Part print with two shaded views. Sizes in mm from the minimum x, y, z corner. Give positions to 0.01 mm unless a question says otherwise; leave off trailing zeros. Write each loop counter-clockwise with the first axis right and the second up, starting at its lowest first coordinate (ties: lowest second). Pieces come first, ordered by that corner, then holes. Notation, with made-up numbers: M -36,62.5 L 11,62.5 A36 ccw 11,101.5 Z; hole C -37,22.25 d6. An arc over 180 degrees is marked long. One line per item, written item: value. Start each with the question number.
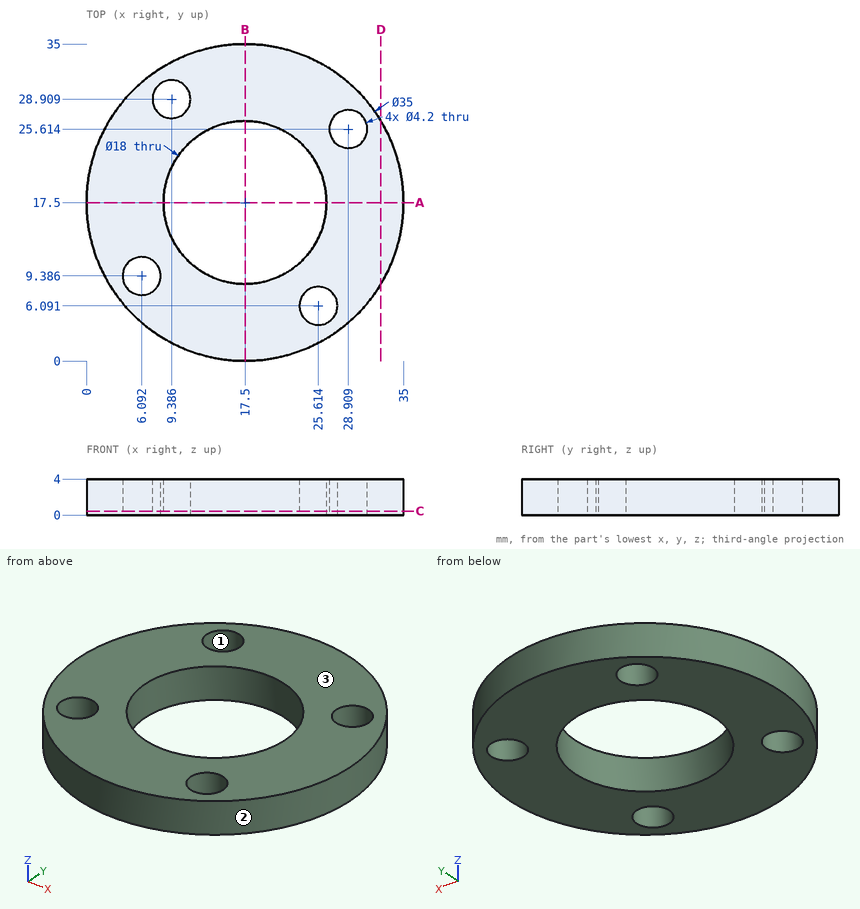
1) Probe line 1 along X through (y, z) = (17.5, 1.95); line 2 along Y through (x, z) = (25, 2.25) (1 decimal); line 3 along X through (y, z) = (10.5, 1.35) (1 decimal). List the from-to ranges inside material, lowest first. Write a range as from..to.
2) Drop flat-ended pins along their axis: P1, Ø3.5, axis at x = 6.09, y = 9.39, coming from the -Z side; P2, Ø10, axis at x = 18.5, y = 22, coming from the -Z side; P3, Ø2, axis at x = 8.5, z = 0.5, coming from the -Y side (1 decimal). Give the stop position or say it passes through.
3) Band-saw the part on D-D (x = 32.5). List the corners of the cut face in (y, z).
4) Band-saw the part on C-C (z = 0.45). List the corners of the cut face in (x, y) (1 decimal).
5) Band-saw the part on A-A (y = 17.5). List the corners of the cut face in (x, z).
6) Mould opens along X. For the marked faces 1, 2 and 3 say: released by +X, released by -X, zero draft, split by the parting line, or undercut.
Model answer:
1. line 1: x = 0..8.5, 26.5..35
1. line 2: y = 1.7..4.1, 8.1..12.5, 22.5..33.3
1. line 3: x = 1.5..4.3, 7.9..11.8, 23.2..33.5
2. P1: passes through
2. P2: stops at z = 0
2. P3: stops at y = 1.9
3. outline: M 8.49,0 L 26.51,0 L 26.51,4 L 8.49,4 Z
4. outline: C 17.5,17.5 d35; hole C 6.1,9.4 d4.2; hole C 9.4,28.9 d4.2; hole C 17.5,17.5 d18; hole C 25.6,6.1 d4.2; hole C 28.9,25.6 d4.2
5. outline: M 0,0 L 8.5,0 L 8.5,4 L 0,4 Z; M 26.5,0 L 35,0 L 35,4 L 26.5,4 Z
6. face 1: undercut
6. face 2: split by the parting line
6. face 3: zero draft
